Could you check a few things on this drawing? It's one solid part, dimensions in mm from its lowest x, y, z. A direction names the side the tool comes from. Round coordinates to 2 decimals unless told otherwise and drop trailing zeros. Write each loop counter-clockwise with the first axis right and the second up, starting at its lowest first coordinate (ties: lowest second). Pieces come first, ordered by that corner, then holes. Notation, with made-up numbers: (35.25, 66.5) -> (74.25, 66.5) arc R25 cw to (74.25, 89.5) -> close; hole circle Ø6 at (-16.75, -15). An arc over 180 degrees is marked (long way). Put each result on its own line as item: value. Start each with the question number.
1) If I drill on line 1 along Z through (x, y) = (5, 3.25); line 2 along X through (y, z) = (6, 11); line 3 along Z through (x, y) = (10.5, 9), over which ranges is the centre line in solid material (lowest first)? Write a range as [from, to].
2) I want a section at A-A, the plane x = 26.5. List the corners of the cut face in (y, z) for me, then the cut area to 3 significant figures.
3) Which directions (+Z, -Z, +X, -X, +Y, -Y) give clear straight access to the entire face, cutting with the end or side of a thin tool? Please do the marked faces 1, 2 and 3.
4) I want a section at B-B, the plane y = 5.5. List the corners of the cut face in (x, z) for me.
5) I want a section at D-D, the plane x = 6. List the corners of the cut face in (y, z) for me.
6) I want a section at C-C, the plane z = 53. List the corners of the cut face in (x, y) for me, then the cut area to 3 significant figures.
7) Will these pins go through, and if not, where does the flat tip stop? P1, Ø5, axis at x = 13, y = 6, coming from the -Z side; P2, Ø3, axis at x = 6, z = 53, coming from the +Y side; P3, Ø2, axis at x = 6.5, y = 5, coming from the +Z side.
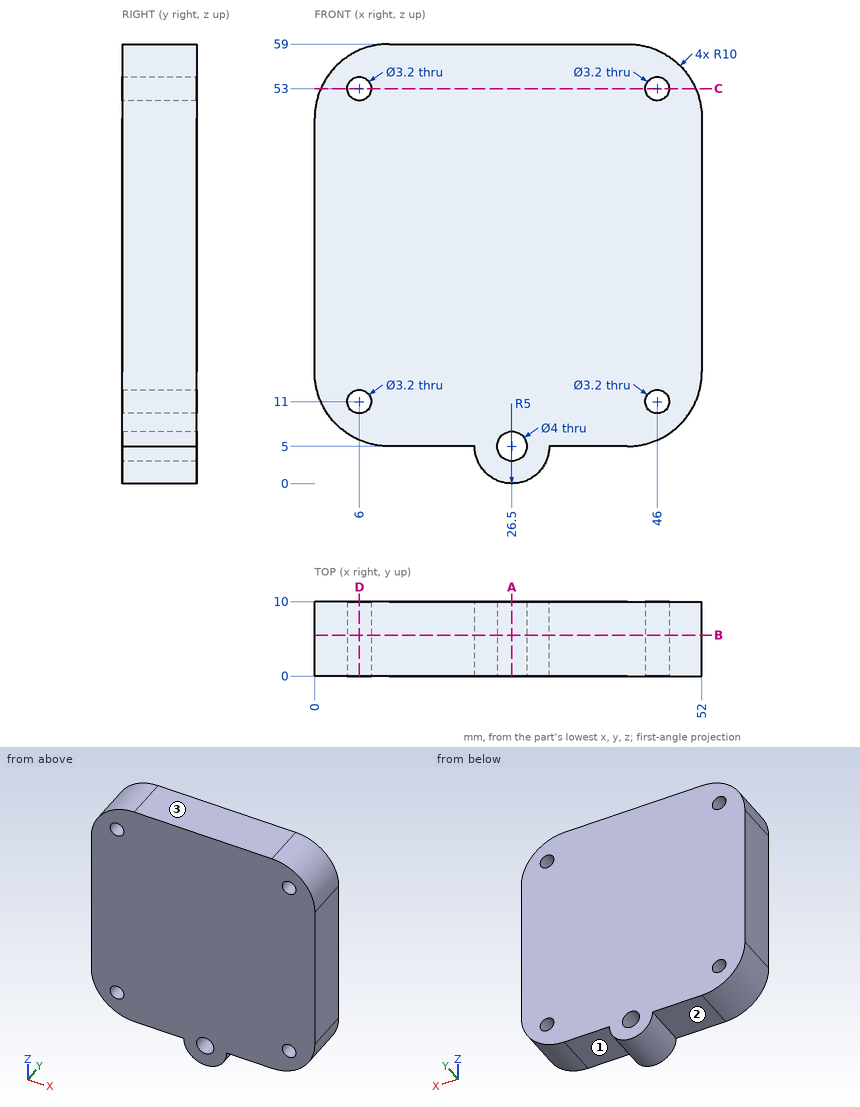
Findings:
1. line 1: z = [6.34, 9.75], [12.25, 51.75], [54.25, 57.66]
1. line 2: x = [0.83, 4.4], [7.6, 44.4], [47.6, 51.17]
1. line 3: z = [5, 59]
2. outline: (0, 0) -> (10, 0) -> (10, 3) -> (0, 3) -> close; (0, 7) -> (10, 7) -> (10, 59) -> (0, 59) -> close
2. area: 550 mm2
3. face 1: -Z, +X, +Y, -Y
3. face 2: -Z, -X, +Y, -Y
3. face 3: +Z, +X, -X, +Y, -Y
4. outline: (0, 15) arc R10 ccw to (10, 5) -> (21.5, 5) arc R5 ccw to (31.5, 5) -> (42, 5) arc R10 ccw to (52, 15) -> (52, 49) arc R10 ccw to (42, 59) -> (10, 59) arc R10 ccw to (0, 49) -> close; hole circle Ø3.2 at (6, 11); hole circle Ø3.2 at (6, 53); hole circle Ø4 at (26.5, 5); hole circle Ø3.2 at (46, 11); hole circle Ø3.2 at (46, 53)
5. outline: (0, 5.83) -> (10, 5.83) -> (10, 9.4) -> (0, 9.4) -> close; (0, 12.6) -> (10, 12.6) -> (10, 51.4) -> (0, 51.4) -> close; (0, 54.6) -> (10, 54.6) -> (10, 58.17) -> (0, 58.17) -> close
6. outline: (0.83, 0) -> (4.4, 0) -> (4.4, 10) -> (0.83, 10) -> close; (7.6, 0) -> (44.4, 0) -> (44.4, 10) -> (7.6, 10) -> close; (47.6, 0) -> (51.17, 0) -> (51.17, 10) -> (47.6, 10) -> close
6. area: 439 mm2
7. P1: stops at z = 5
7. P2: passes through
7. P3: stops at z = 58.68
